Source: three-view drawing plus pictorial views. Frame: mm from the lowest corner of the part. Give positions to 0.01 mm unless a question says otherwise; leave off trailing zeros. Loops run counter-clockwise (first coordinate to the right, second up) from the corner with the lowest first, then second, coordinate; pieces in that order, holes last. Notation, with made-up numbers: (79, 57.25) -> (129, 57.25) arc R15 ccw to (129, 78.25) -> close; hole circle Ø6 at (12.25, 43). An arc over 180 degrees is marked (long way). Answer as a JSON object with one key per item and string values. Group by question number.
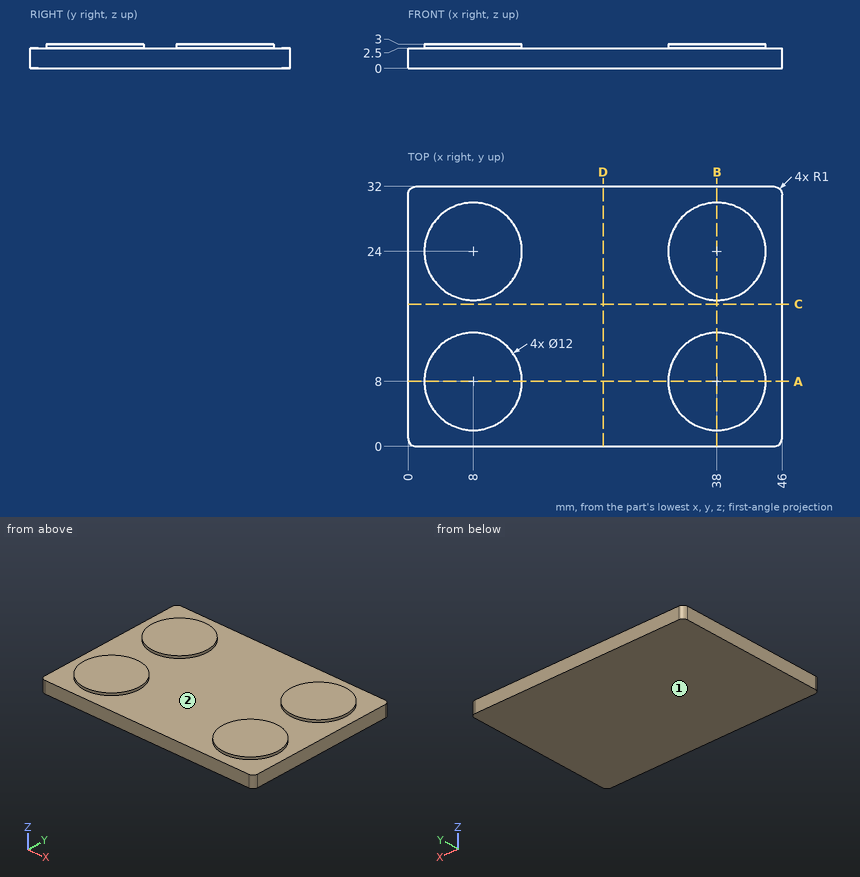
Q1. Section D-D on x = 24. Return the cut outline in (y, z), then the cut area to 3 significant figures.
Q2. Section A-A on y = 8. Return the cut outline in (x, z).
Q3. Section C-C on y = 17.5. Return the cut outline in (x, z), then the cut area to 3 significant figures.
Q4. Pull-direction query (X, two-part tool) for the marked faces 1 and 2; classes: +X half, -X half, draft (parallel to the pull), parting line (faces both ways), or undercut.
Q5. Section B-B on x = 38. Return the cut outline in (y, z).
Q6. Ray query, probe 1 along Z at (x, y) = (26.5, 10); probe 2 along Y at (x, z) = (38.5, 2.7); probe 3 along X at (y, z) = (4, 2.55). Return the intervals inside material, ascending.
Numbers:
{
 "1": {"outline": "(0, 0) -> (32, 0) -> (32, 2.5) -> (0, 2.5) -> close", "area": "80.0 mm²"},
 "2": {"outline": "(0, 0) -> (46, 0) -> (46, 2.5) -> (44, 2.5) -> (44, 3) -> (32, 3) -> (32, 2.5) -> (14, 2.5) -> (14, 3) -> (2, 3) -> (2, 2.5) -> (0, 2.5) -> close"},
 "3": {"outline": "(0, 0) -> (46, 0) -> (46, 2.5) -> (0, 2.5) -> close", "area": "115 mm²"},
 "4": {"face 1": "draft", "face 2": "undercut"},
 "5": {"outline": "(0, 0) -> (32, 0) -> (32, 2.5) -> (30, 2.5) -> (30, 3) -> (18, 3) -> (18, 2.5) -> (14, 2.5) -> (14, 3) -> (2, 3) -> (2, 2.5) -> (0, 2.5) -> close"},
 "6": {"probe 1": "z = 0 to 2.5", "probe 2": "y = 2.02 to 13.98, 18.02 to 29.98", "probe 3": "x = 3.53 to 12.47, 33.53 to 42.47"}
}
